Verification items for this drawing (mm, ordinates from the low corner). Round coordinates to 2 decimals unless told otherwise and drop trailing zeros. Order: outer loops, then holes, each group sorted by start corner. A loop starts at its lowest first (then second) coordinate and runs counter-clockwise, first axis right, second up. Notation, with made-up numbers: (25, -1.5) - (43, -1.5) arc R20 ccw to (43, 11.5) - close; hole circle Ø10 at (56, -18). An arc over 180 degrees is marked (long way). Use a Markdown table: item, result. Add a question column.
(1) Section check A-A on x = 9. Record the boundary of the cut face in (y, z).
(2) Section check B-B on z = 8.5. Record the boundary of the cut face in (x, y).
(3) Section check D-D on y = 24. Record the boundary of the cut face in (x, z).
(4) Section check C-C on x = 4.5. Record the boundary of the cut face in (y, z) (1 decimal).
(5) Gauge pin test, flat ends, axial feed: P1, Ø3, axis at x = 21.5, y = 21.5, coming from the +Z side; P2, Ø5.5, axis at x = 5, y = 5, coming from the +Z side; P3, Ø15, axis at x = 20, y = 14, coming from the -Z side; P4, Ø2, axis at y = 30.5, z = 4.5, coming from the -X side. Record the tip position at first contact, or that the pin passes through.
(6) Thickness scan on line 1 along Y through (x, z) = (5, 5.5); line 2 along X through (y, z) = (6.5, 13.25) (1 decimal). Record the ranges inside material, lowest first. Write a range as [from, to].
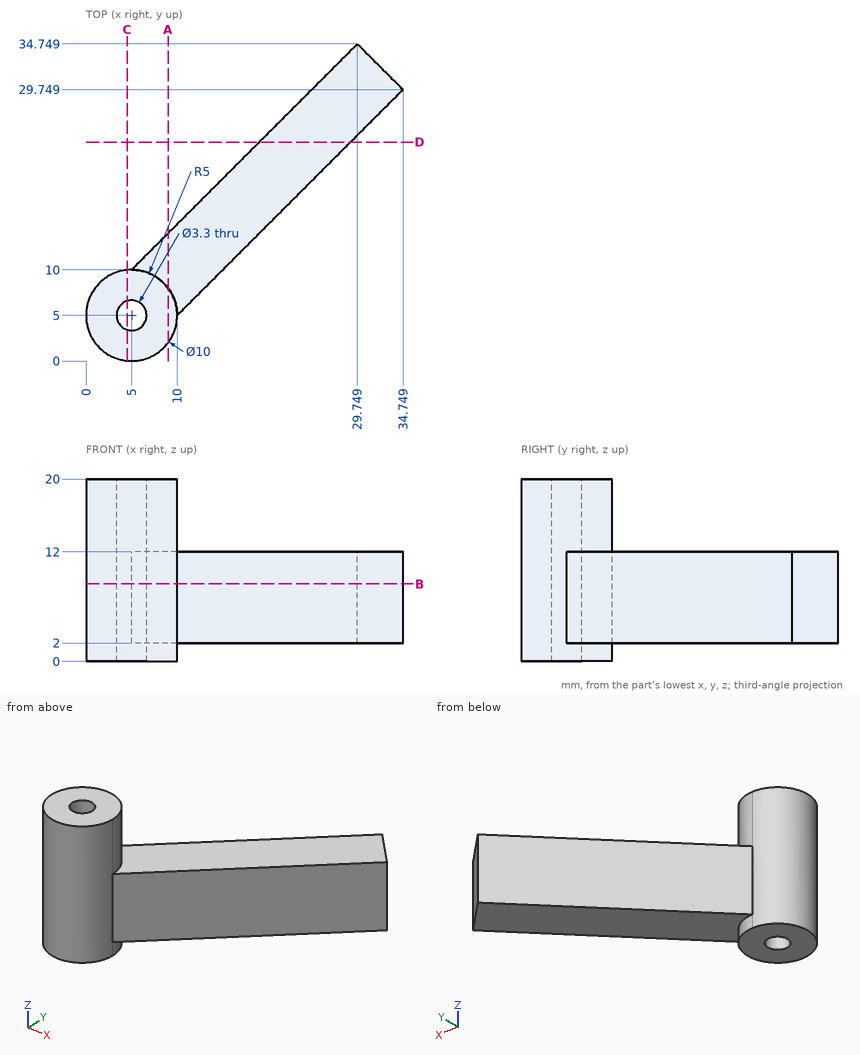
Check sheet entries:
| question | item | result |
|---|---|---|
| 1 | outline | (2, 0) - (8, 0) - (8, 2) - (14, 2) - (14, 12) - (8, 12) - (8, 20) - (2, 20) - close |
| 2 | outline | (5, 10) arc R5 ccw (long way) to (10, 5) - (34.75, 29.75) - (29.75, 34.75) - close; hole circle Ø3.3 at (5, 5) |
| 3 | outline | (19, 2) - (29, 2) - (29, 12) - (19, 12) - close |
| 4 | outline | (0, 0) - (3.4, 0) - (3.4, 20) - (0, 20) - close; (6.6, 0) - (10, 0) - (10, 20) - (6.6, 20) - close |
| 5 | P1 | stops at z = 12 |
| 5 | P2 | stops at z = 20 |
| 5 | P3 | stops at z = 2 |
| 5 | P4 | stops at x = 24.5 |
| 6 | line 1 | y = [0, 3.35], [6.65, 10] |
| 6 | line 2 | x = [0.2, 4.3], [5.7, 9.8] |
